Can you work these out from the drawing? Everything is in mm from the part's minimum corner. Give positions to 0.01 mm unless a question says otherwise; leave off trailing zeros. Write each loop counter-clockwise with the first axis right and the second up, starting at its lowest first coordinate (ties: lowest second). Pieces come first, ordered by that corner, then holes. Notation, with made-up numbers: (24.5, 86) - (42.5, 86) arc R20 ccw to (42.5, 99) - close; hole circle Ø5 at (35, -33). An arc over 180 degrees is marked (long way). Answer in a Markdown table with one row per item.
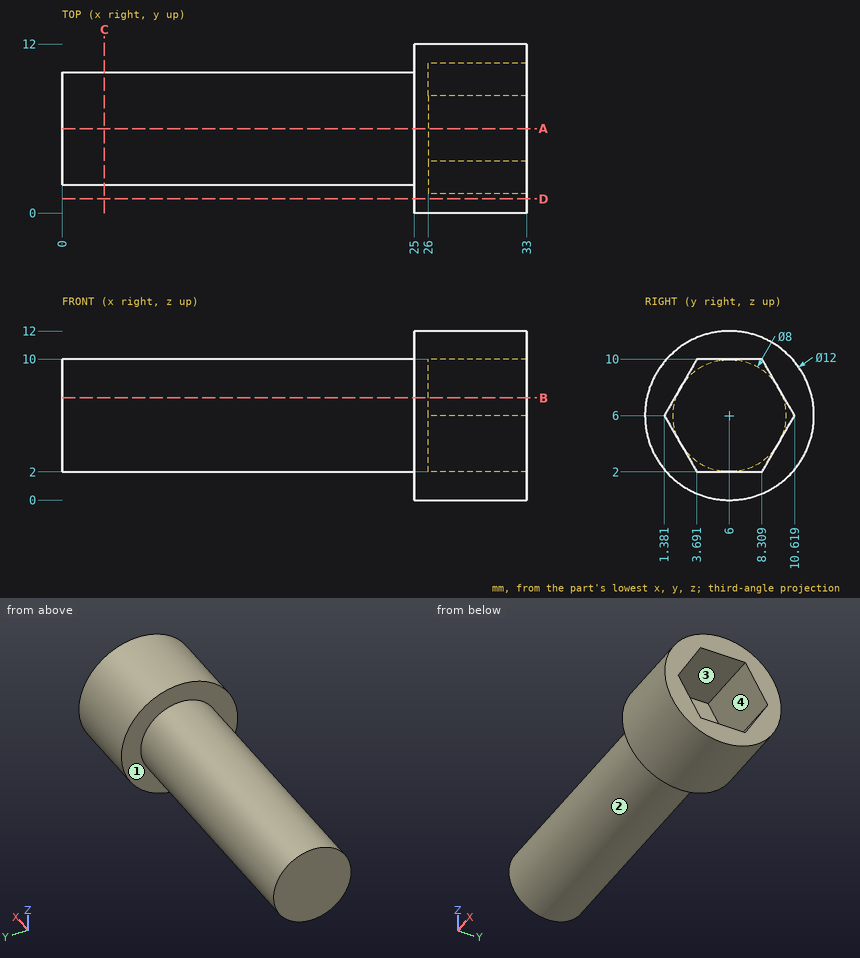
1) Imagine slicing it at D-D (y = 1). List the corners of the cut face in (x, z) for me.
Check values:
| item | result |
|---|---|
| outline | (25, 2.68) - (33, 2.68) - (33, 9.32) - (25, 9.32) - close |
2) We'd pull the mould along Y, two halves only. Please class the marked faces 1, 2, 3 and 4: +Y half, -Y half, draft (parallel to the pull), parting line (faces both ways), or undercut.
Check values:
| item | result |
|---|---|
| face 1 | draft |
| face 2 | parting line |
| face 3 | undercut |
| face 4 | undercut |
3) Imagine slicing it at A-A (y = 6). List the corners of the cut face in (x, z) for me, then the cut area to 3 significant figures.
Check values:
| item | result |
|---|---|
| outline | (0, 2) - (25, 2) - (25, 0) - (33, 0) - (33, 2) - (26, 2) - (26, 10) - (33, 10) - (33, 12) - (25, 12) - (25, 10) - (0, 10) - close |
| area | 240 mm2 |
4) Imagine slicing it at C-C (x = 3). List the corners of the cut face in (y, z) for me.
Check values:
| item | result |
|---|---|
| outline | circle Ø8 at (6, 6) |
5) Will these pins go through, and if not, where does the flat tip stop? P1, Ø2, axis at x = 24.5, z = 3, coming from the +Y side; P2, Ø5, axis at x = 18.5, z = 5.5, coming from the +Y side; P3, Ø4, axis at y = 4.5, z = 5.5, coming from the +X side.
Check values:
| item | result |
|---|---|
| P1 | stops at y = 11.61 |
| P2 | stops at y = 10 |
| P3 | stops at x = 26 |
6) Imagine slicing it at B-B (z = 7.25). List the corners of the cut face in (x, y) for me, then the cut area to 3 significant figures.
Check values:
| item | result |
|---|---|
| outline | (0, 2.2) - (25, 2.2) - (25, 0.13) - (33, 0.13) - (33, 2.1) - (26, 2.1) - (26, 9.9) - (33, 9.9) - (33, 11.87) - (25, 11.87) - (25, 9.8) - (0, 9.8) - close |
| area | 229 mm2 |
7) If I drill on line 1 (X direction, y = 10, z = 8.25); line 2 (X direction, y = 6.5, z = 5.25); line 3 (Y direction, x = 24.5, z = 5.75), over which ranges is the centre line in solid material (lowest first)?
Check values:
| item | result |
|---|---|
| line 1 | x = 25 to 33 |
| line 2 | x = 0 to 26 |
| line 3 | y = 2.01 to 9.99 |
